Solid Edge part; units mm, degrees
sketch "Sketch1" plane through (0, 0, 0) normal (0, 0, 1) x (1, 0, 0)
  circle A0 centre (0, 0) radius 16.5
  line L0 (-21, 21) -> (21, 21)
  line L1 (21, 21) -> (21, -21)
  line L2 (21, -21) -> (-21, -21)
  line L3 (-21, -21) -> (-21, 21)
extrude "Protrusion1" add sketch "Sketch1" along normal blind 11
sketch "Sketch2" plane through (0, 0, 0) normal (0, 0, -1) x (0, 1, 0)
  circle A0 centre (-15.5, 15.5) radius 1.2295
  circle A1 centre (15.5, 15.5) radius 1.2295
  circle A2 centre (-15.5, -15.5) radius 1.2295
  circle A3 centre (15.5, -15.5) radius 1.2295
extrude "ExtrudedCutout_1" cut sketch "Sketch2" against normal blind 24
sketch "Sketch3" plane through (0, 0, 0) normal (0, 0, -1) x (0, 1, 0)
  circle A0 centre (74.8245, 0) radius 11.2
  line L0 (21, 21) -> (21, -21)
  line L1 (89.3061, -21) -> (21, -21)
  line L2 (89.3061, 14.6519) -> (89.3061, -21)
  line L3 (60.6266, 14.6519) -> (89.3061, 14.6519)
  line L4 (21, 21) -> (60.6266, 14.6519)
extrude "Protrusion2" add sketch "Sketch3" against normal up to vertex (7.2 mm away)
sketch "Sketch4" plane through (0, 55.1531, 7.2) normal (0, 0, 1) x (0, 1, 0)
  line L0 (-30.0866, 16.7943) -> (0.1278, 16.7943)
  line L1 (0.1278, 16.7943) -> (0.1278, -10.1482)
  line L2 (0.1278, -10.1482) -> (-30.0866, -14.9885)
  line L3 (-30.0866, -14.9885) -> (-30.0866, 16.7943)
extrude "ExtrudedCutout_3" cut sketch "Sketch4" against normal blind 194
sketch "Sketch5" plane through (0, 55.1531, 7.2) normal (0, 0, 1) x (0, 1, 0)
  circle A0 centre (19.6714, 0) radius 14.4816
  circle A1 centre (19.6714, 0) radius 4.75
extrude "ExtrudedProtrusion_3" add sketch "Sketch5" along normal blind 3
sketch "Sketch6" plane through (14.6519, 74.9664, 3.6) normal (1, 0, 0) x (0, 1, 0)
  line L0 (-14.6235, 3.6) -> (14.3398, 3.6)
  line L1 (14.3398, 3.6) -> (14.3398, 22)
  line L2 (14.3398, 22) -> (-14.6235, 22)
  line L3 (-14.6235, 22) -> (-14.6235, 3.6)
  line L4 (-1.5561, 14.2142) -> (-0.1419, 15.6284)
  line L5 (-0.1419, 15.6284) -> (1.2723, 14.2142)
  arc A0 (1.2723, 14.2142) -> (-1.5561, 14.2142) centre (-0.1419, 12.8) cw
extrude "Protrusion3" add sketch "Sketch6" against normal up to vertex (35.6519 mm away)
sketch "Sketch7" plane through (0, 34.1531, 0) normal (0, 0, -1) x (1, 0, 0)
  circle A0 centre (0, -40.6714) radius 2.5
extrude "ExtrudedCutout_4" cut sketch "Sketch7" against normal blind 682
sketch "Sketch8" plane through (-3.1741, 74.8245, 25.6) normal (0, 0, 1) x (0, -1, 0)
  circle A0 centre (0, 3.1741) radius 11.2
extrude "ExtrudedCutout_5" cut sketch "Sketch8" against normal blind 21.6
Check sheet for the modelled part. Datum: model origin and axes. Units: mm. A direction names the side the tool comes from. Round coordinates to 2 decimals unless told otherwise and drop trailing zeros. Order: outer loops, then holes, each group sorted by start corner. A loop starts at its lowest first (then second) coordinate and runs counter-clockwise, first axis right, second up. Notation, with made-up numbers: M -33,3 L -9,3 A32 cw -9,42 Z; hole C 81.5,76.25 d8. An arc over 180 degrees is marked long. Answer in a Markdown table with one row per item.
(1) Set-up check for faces 4 (the flat face through (14.652, 75, 13)), 5 (the flat face through (0, 21, 9)), 6 (the flat face through (-11, 72, 25.6)), 7 (the flat face through (-16.794, 40, 4)): record each of +Z, -Z, +X, -X, +Y, -Y from which the full face is reachable in a straight line by a thin tool's end or side.
Findings:
| item | result |
|---|---|
| face 4 | +Z, -Z, +X, +Y |
| face 5 | +Z, +X, -X |
| face 6 | +Z, +X, -X, +Y, -Y |
| face 7 | +Z, -Z |
(2) Gauge pin test, flat ends, axial feed: pin 1 (9 mm diameter, centred on x = -2, z = 17, fed in from -Y); pin 2 (1.5 mm diameter, centred on y = 37.5, z = 5, fed in from +X); pin 3 (20 mm diameter, centred on x = 4.5, y = 34.5, fed in from +Z). Record the tip position at first contact, or that the pin passes through.
Findings:
| item | result |
|---|---|
| pin 1 | stops at y = 60.34 |
| pin 2 | stops at x = 18.48 |
| pin 3 | stops at z = 7.2 |
(3) Section check C-C on y = 36.5. Record the boundary of the cut face in (x, z).
Findings:
| item | result |
|---|---|
| outline | M -21,0 L -16.79,0 L -16.79,7.2 L -21,7.2 Z; M 13.16,0 L 18.52,0 L 18.52,7.2 L 13.16,7.2 Z |
(4) Material ranges on line 1 along Y through (x, z) = (8.5, 10.5); line 2 along Y through (x, z) = (3, 9.75); line 3 along Y through (x, z) = (-15.75, 16.4), recorded low to high. Write a range as from..to.
Findings:
| item | result |
|---|---|
| line 1 | y = -21..-14.14, 14.14..21, 60.34..67.53, 82.12..89.31 |
| line 2 | y = -21..-16.22, 16.22..21, 60.34..64.03, 85.62..89.31 |
| line 3 | y = 60.34..72.82, 76.82..89.31 |
(5) Section check A-A on z = 8.25. Record the boundary of the cut face in (x, y), plus the area to 3 significant figures.
Findings:
| item | result |
|---|---|
| outline | M -21,-21 L 21,-21 L 21,21 L -21,21 Z; M -21,60.34 L 14.65,60.34 L 14.65,89.31 L -21,89.31 Z; hole C -15.5,-15.5 d2.46; hole C -15.5,15.5 d2.46; hole C 0,0 d33; hole C 0,74.82 d22.4; hole C 15.5,-15.5 d2.46; hole C 15.5,15.5 d2.46 |
| area | 1,530 mm^2 |
(6) Draft check along X on faces 1 (the flat face through (-21, 46, 7)), 2 (the cylindrical face through (15.24, 6.32, 5.42)), 3 (the flat face through (0, -21, 5)). Enter one of: +X half, -X half, draft (parallel to the pull), parting line (faces both ways), or undercut.
Findings:
| item | result |
|---|---|
| face 1 | -X half |
| face 2 | undercut |
| face 3 | draft |
(7) Section check D-D on z = 23. Record the boundary of the cut face in (x, y).
Findings:
| item | result |
|---|---|
| outline | M -21,60.34 L 14.65,60.34 L 14.65,89.31 L -21,89.31 Z; hole C 0,74.82 d22.4 |
(8) Section check B-B on x = -15.5. Give the number of separate pieces and of enclosed holes in the cut face, plus the area to 3 significant figures.
Findings:
| item | result |
|---|---|
| separate pieces | 5 |
| enclosed holes | 1 |
| area | 1,080 mm^2 |
